Can you work these out from the drawing? Everything is in mm from the part's minimum corner. Round coordinates to 2 decimals unless told otherwise and drop trailing zeros. Loops run counter-clockwise (first coordinate to the right, second up) from the corner with the lowest first, then second, coordinate; pieces in that order, holes last. Notation, with made-up numbers: M 60,8.25 L 75,8.25 A20 ccw 75,25.25 Z; hole C -30,-4 d1. An arc over 180 degrees is marked long. Use a Markdown table: item, result.
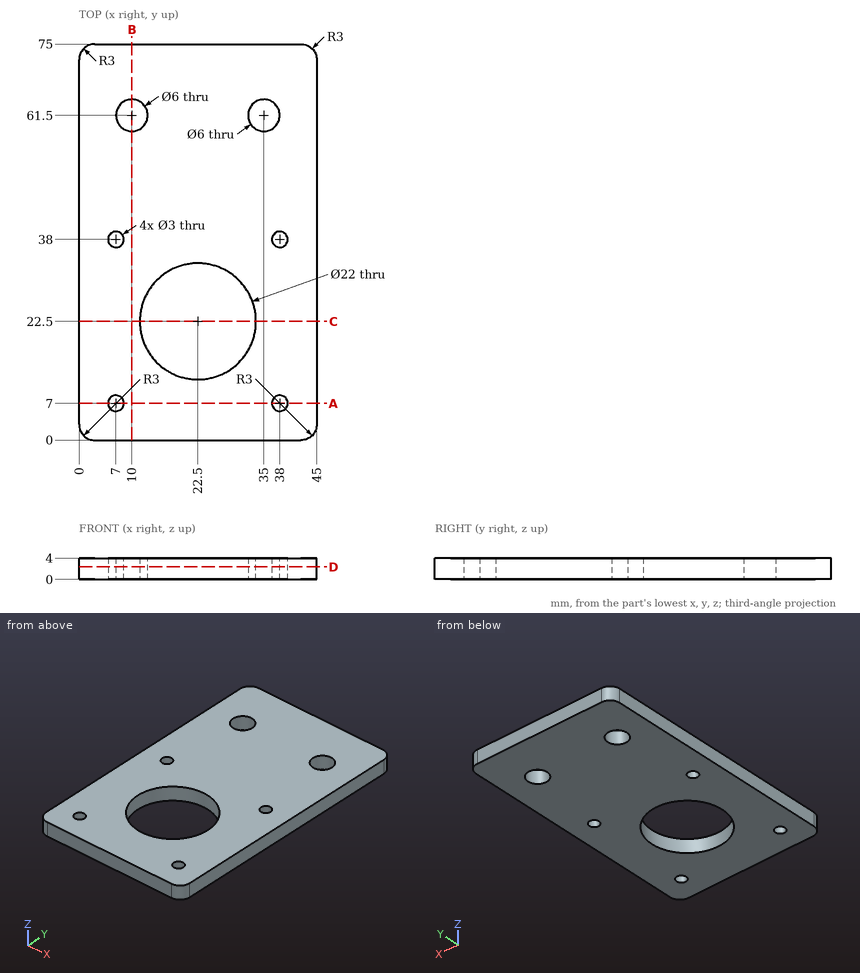
1. I need wall thicknesses on probe 1 along X at (y, z) = (39, 3.25); probe 2 along Y at (x, z) = (35, 0.75); probe 3 along X at (y, z) = (59, 1.9). Which ranges of each line are inside material? Lowest first, please. Write a range as from..to.
Answer sheet:
| item | result |
|---|---|
| probe 1 | 0..5.88, 8.12..36.88, 39.12..45 |
| probe 2 | 0..58.5, 64.5..75 |
| probe 3 | 0..8.34, 11.66..33.34, 36.66..45 |
2. Imagine slicing it at A-A, the plane y = 7. Write out the boundary of the cut face in (x, z), then the cut area to 3 significant figures.
Answer sheet:
| item | result |
|---|---|
| outline | M 0,0 L 5.5,0 L 5.5,4 L 0,4 Z; M 8.5,0 L 36.5,0 L 36.5,4 L 8.5,4 Z; M 39.5,0 L 45,0 L 45,4 L 39.5,4 Z |
| area | 156 mm2 |
3. Imagine slicing it at D-D, the plane z = 2.35. Write out the boundary of the cut face in (x, y).
Answer sheet:
| item | result |
|---|---|
| outline | M 0,3 A3 ccw 3,0 L 42,0 A3 ccw 45,3 L 45,72 A3 ccw 42,75 L 3,75 A3 ccw 0,72 Z; hole C 7,7 d3; hole C 7,38 d3; hole C 10,61.5 d6; hole C 22.5,22.5 d22; hole C 35,61.5 d6; hole C 38,7 d3; hole C 38,38 d3 |
4. Imagine slicing it at B-B, the plane x = 10. Write out the boundary of the cut face in (y, z).
Answer sheet:
| item | result |
|---|---|
| outline | M 0,0 L 58.5,0 L 58.5,4 L 0,4 Z; M 64.5,0 L 75,0 L 75,4 L 64.5,4 Z |
5. Imagine slicing it at C-C, the plane y = 22.5. Write out the boundary of the cut face in (x, z).
Answer sheet:
| item | result |
|---|---|
| outline | M 0,0 L 11.5,0 L 11.5,4 L 0,4 Z; M 33.5,0 L 45,0 L 45,4 L 33.5,4 Z |
